```python
from build123d import *

# Parameters (mm, degrees)
EXTRUDE_1_DEPTH          = 240
CUT_EXTRUDE_3_DEPTH      = 326.109212419
CUT_EXTRUDE_3_DEPTH_BACK = 326.109212419
EXTRUDE_3_DEPTH          = 3
SKETCH_11_W              = 50
SKETCH_11_H              = 186
EXTRUDE_5_DEPTH          = 40
CUT_EXTRUDE_4_DEPTH      = 183
SKETCH_13_R              = 10
SKETCH_13_R_2            = 3
SKETCH_13_R_3            = 5.2
CUT_EXTRUDE_5_DEPTH      = 187
SKETCH_16_W              = 44
SKETCH_16_H              = 20
CUT_EXTRUDE_6_DEPTH      = 3


with BuildPart() as part:
    # 草图2 → 凸台-拉伸1 (new body)
    with BuildSketch(Plane(origin=(0, 0, 0), x_dir=(1, 0, 0), z_dir=(0, 1, 0))):
        with BuildLine():
            Line((0, 0), (200, 0))
            ThreePointArc((200, 0), (100, 100), (0, 0))
        make_face()
    extrude(amount=EXTRUDE_1_DEPTH)

    # 草图4 → 切除-拉伸3 (cut, two sides: drawn at the far end of the back side and taken through both)
    with BuildSketch(Plane(origin=(0, 4, 0), x_dir=(1, 0, 0), z_dir=(0, 1, 0)).offset(-CUT_EXTRUDE_3_DEPTH_BACK)):
        with BuildLine():
            Line((3, 3), (197, 3))
            ThreePointArc((197, 3), (100, 96.979861709), (3, 3))
        make_face()
    extrude(amount=CUT_EXTRUDE_3_DEPTH + CUT_EXTRUDE_3_DEPTH_BACK, mode=Mode.SUBTRACT)

    # 草图10 → 凸台-拉伸3 (add)
    with BuildSketch(Plane(origin=(0, 0, 0), x_dir=(1, 0, 0), z_dir=(0, 1, 0))):
        with BuildLine():
            Line((3, 3), (197, 3))
            ThreePointArc((197, 3), (100, 96.979861709), (3, 3))
        make_face()
    extrude(amount=EXTRUDE_3_DEPTH)

    # 草图11 → 凸台-拉伸5 (add)
    with BuildSketch(Plane(origin=(0, 0, -3), x_dir=(-1, 0, 0), z_dir=(0, 0, -1))):
        with Locations((-139.082312279, 147)):
            Rectangle(SKETCH_11_W, SKETCH_11_H)
    extrude(amount=EXTRUDE_5_DEPTH)

    # 草图12 → 切除-拉伸4 (cut)
    with BuildSketch(Plane(origin=(0, 240, 0), x_dir=(1, 0, 0), z_dir=(0, 1, 0))):
        Polygon((117.082312279, 3), (117.082312279, 40), (128.082312279, 40), (131.082312279, 40), (161.082312279, 40), (161.082312279, 3), (131.082312279, 3), (128.082312279, 3), align=None)
    extrude(amount=-CUT_EXTRUDE_4_DEPTH, mode=Mode.SUBTRACT)

    # 草图13 → 切除-拉伸5 (cut)
    with BuildSketch(Plane(origin=(0, 240, 0), x_dir=(1, 0, 0), z_dir=(0, 1, 0))):
        with Locations(Location((144.331422693, 21.213361888, 0), (0, 0, 270))):
            Circle(SKETCH_13_R)
        with Locations(Location((123.835336357, 21.213361888, 0), (0, 0, 270))):
            Circle(SKETCH_13_R_2)
        with Locations(Location((123.835336357, 10.323097486, 0), (0, 0, 270))):
            Circle(SKETCH_13_R_3)
        with Locations(Location((123.835336357, 33.165384847, 0), (0, 0, 270))):
            Circle(SKETCH_13_R_3)
    extrude(amount=-CUT_EXTRUDE_5_DEPTH, mode=Mode.SUBTRACT)

    # 草图16 → 切除-拉伸6 (cut)
    with BuildSketch(Plane.XY):
        with Locations((139.082312279, 190)):
            Rectangle(SKETCH_16_W, SKETCH_16_H)
    extrude(amount=-CUT_EXTRUDE_6_DEPTH, mode=Mode.SUBTRACT)


solid = part.part
```
Source: CAD feature listing. Evaluate the final solid. Frame: model axes, mm. A direction names the side the tool comes from. Round coordinates to 2 decimals unless told otherwise and drop trailing zeros. Loops run counter-clockwise (first coordinate to the right, second up) from the corner with the lowest first, then second, coordinate; pieces in that order, holes last.
1. Section query D-D on x = 141. Output: boundary loops of the cut face in (y, z).
2. Section query B-B on y = 109. Output: boundary loops of the cut face in (x, z), and give its area (3 significant figures).
3. Section query A-A on y = 184. Output: boundary loops of the cut face in (x, z).
4. Access query for faces 1 (the flat face through (99, 118, 0)), 2 (the flat face through (164.082, 146, -23)). Directions: +Z, -Z, +X, -X, +Y, -Y. A direction counts if a zero-diameter tool reaches every point of the face in a straight line with its end or side. Return the directions, or none.
5. Section query C-C on x = 100. Output: boundary loops of the cut face in (y, z).
6. Ray query, L1, parallel to X at y = 101.5, z = -15; L2, parallel to X at y = 97, z = -3.5; L3, parallel to Z at x = 98.5, y = 54. Return the intervals inside material, ascending.
7. Contact query for flat-ended pins moving along their axis: pin 1 (3.5 mm diameter, centred on x = 123.84, z = -21.21, fed in from +Y); pin 2 (1.5 mm diameter, centred on x = 179.5, y = 132, fed in from +Z); pin 3 (1 mm diameter, centred on x = 137, y = 64.5, fed in from -Z); pin 4 (8 mm diameter, centred on y = 52.5, z = -50, fed in from +X). Output: stop coordinate, or through.
8. Mould query, pull axis X, two halves, no side actions, for faces 3 (the cylindrical face through (102.199, 118.32, -99.976)), 4 (the flat face through (114.3, 240, -35.4)), 5 (the flat face through (77, 120, -3)). Classes: released by +X, released by -X, zero draft, split by the parting line, or undercut.
Answers below:
1. outline: (0, -91.21) - (240, -91.21) - (240, -87.89) - (3, -87.89) - (3, -3) - (54, -3) - (54, -11.78) - (57, -11.78) - (57, -3) - (180, -3) - (180, 0) - (0, 0) - close; (54, -43) - (240, -43) - (240, -40) - (57, -40) - (57, -30.64) - (54, -30.64) - close; (200, -3) - (240, -3) - (240, 0) - (200, 0) - close
2. outline: (0, 0) arc R100 ccw to (200, 0) - close; hole (3, -3) arc R97.05 ccw to (197, -3) - (164.08, -3) - (164.08, -43) - (114.08, -43) - (114.08, -3) - close; hole (117.08, -40) - (161.08, -40) - (161.08, -3) - (117.08, -3) - close
2. area: 1,880 mm2
3. outline: (0, 0) arc R100 ccw to (200, 0) - (161.08, 0) - (161.08, -40) - (117.08, -40) - (117.08, 0) - close; hole (3, -3) arc R97.05 ccw to (197, -3) - (164.08, -3) - (164.08, -43) - (114.08, -43) - (114.08, -3) - close
4. face 1: +Z, +X, -X, +Y, -Y
4. face 2: +Y
5. outline: (0, -100) - (240, -100) - (240, -96.98) - (3, -96.98) - (3, -3) - (240, -3) - (240, 0) - (0, 0) - close
6. L1: x = 1.13 to 4.13, 114.08 to 117.08, 161.08 to 164.08, 195.87 to 198.87
6. L2: x = 0.06 to 3.02, 114.08 to 117.08, 161.08 to 164.08, 196.98 to 199.94
6. L3: z = -99.99 to -96.97, -3 to 0
7. pin 1: stops at y = 3
7. pin 2: stops at z = 0
7. pin 3: stops at z = -93.1
7. pin 4: stops at x = 188.79
8. face 3: split by the parting line
8. face 4: zero draft
8. face 5: undercut
